from build123d import *

# Parameters (mm, degrees)
F0_W     = 38.354
F0_H     = 38.354
F0_W_2   = 28.829
F0_H_2   = 28.829
F1_DEPTH = 12.7
F2_R     = 5.969
F3_R     = 3.175
F4_R     = 3.81
F5_DEPTH = 43.688


with BuildPart() as f1:
    # F0 (on Front) → F1 (new body, symmetric)
    with BuildSketch(Plane.XZ):
        Rectangle(F0_W, F0_H)
        Rectangle(F0_W_2, F0_H_2, mode=Mode.SUBTRACT)
    extrude(amount=F1_DEPTH, both=True)

    # F2
    f2_edges = [f1.edges().sort_by_distance(p)[0] for p in [
        (-19.177, 0, 19.177),
        (19.177, 0, 19.177),
        (19.177, 0, -19.177),
        (-19.177, 0, -19.177),
    ]]
    fillet(f2_edges, radius=F2_R)

    # F3
    f3_edges = [f1.edges().sort_by_distance(p)[0] for p in [
        (-14.4145, 0, 14.4145),
        (14.4145, 0, 14.4145),
        (14.4145, 0, -14.4145),
        (-14.4145, 0, -14.4145),
    ]]
    fillet(f3_edges, radius=F3_R)

    # F4 (on face) → F5 (cut)
    with BuildSketch(Plane.XY.offset(19.177)):
        Circle(F4_R)
    extrude(amount=-F5_DEPTH, mode=Mode.SUBTRACT)


solid = f1.part
Can you work these out from the model? Positions are in its coordinate system, mm. A direction names the side the tool comes from. Give positions to 0.01 mm unless a question says otherwise; leave off trailing zeros. Write each loop counter-clockwise with the first axis right and the second up, starting at its lowest first coordinate (ties: lowest second). Pieces come first, ordered by that corner, then holes. Notation, with made-up numbers: M 62,26 L 89,26 A10 ccw 89,43 Z; hole C 33.5,18.5 d4. An arc over 180 degrees is marked long. Answer in a Markdown table with one row per item. Add a question column.
Item 1: Imagine slicing it at C-C, the plane z = 3. Write out the boundary of the cut face in (x, y).
Item 2: Imagine slicing it at D-D, the plane x = 0. Write out the boundary of the cut face in (y, z).
Item 3: On a 3-axis mill with a long thin cutter (end or side, diameter ignored), from which of +Z, -Z, +X, -X, +Y, -Y can I reach the whole of each face in a straight line? I mean faces 1 (the cylindrical face through (13.51, 0.18, 13.46)), 2 (the flat face through (-3, 3, 19.177)). Say none if no direction works.
Item 4: Please list where these lines run through material, in increasing order: L1, parallel to Y at x = 0, z = -15.95; L2, parallel to Z at x = -7, y = -10.5.
Item 5: We'd pull the mould along X, two halves only. Please class faces 3 (the cylindrical face through (-0.83, -3.72, -16.76)), 4 (the cylindrical face through (-0.83, -3.72, 16.83)), 5 (the cylindrical face through (-17.475, -0.178, -17.382)), 6 (the cylindrical face through (17.475, 0.178, 17.382)): released by +X, released by -X, zero draft, split by the parting line, or undercut.
Item 6: Imagine slicing it at B-B, the plane x = 7. Write out the boundary of the cut face in (y, z), plus the area to 3 significant figures.
Item 7: For pin 1 Ø6 at (x, y) = (0, 0) entering from +Z, with a flat end and sliding along its axis, tell me the tip position at first contact or that it passes through.
Evaluation:
| question | item | result |
|---|---|---|
| 1 | outline | M -19.18,-12.7 L -14.41,-12.7 L -14.41,12.7 L -19.18,12.7 Z; M 14.41,-12.7 L 19.18,-12.7 L 19.18,12.7 L 14.41,12.7 Z |
| 2 | outline | M -12.7,-19.18 L -3.81,-19.18 L -3.81,-14.41 L -12.7,-14.41 Z; M -12.7,14.41 L -3.81,14.41 L -3.81,19.18 L -12.7,19.18 Z; M 3.81,-19.18 L 12.7,-19.18 L 12.7,-14.41 L 3.81,-14.41 Z; M 3.81,14.41 L 12.7,14.41 L 12.7,19.18 L 3.81,19.18 Z |
| 3 | face 1 | +Y, -Y |
| 3 | face 2 | +Z, +X, -X, +Y, -Y |
| 4 | L1 | y = -12.7 to -3.81, 3.81 to 12.7 |
| 4 | L2 | z = -19.18 to -14.41, 14.41 to 19.18 |
| 5 | face 3 | undercut |
| 5 | face 4 | undercut |
| 5 | face 5 | released by -X |
| 5 | face 6 | released by +X |
| 6 | outline | M -12.7,-19.18 L 12.7,-19.18 L 12.7,-14.41 L -12.7,-14.41 Z; M -12.7,14.41 L 12.7,14.41 L 12.7,19.18 L -12.7,19.18 Z |
| 6 | area | 242 mm² |
| 7 | pin 1 | passes through |
